Part model, mm, in its own coordinate system. A direction names the side the tool comes from. Round coordinates to 2 decimals unless told otherwise and drop trailing zeros. Write each loop counter-clockwise with the first axis right and the second up, starting at its lowest first coordinate (ties: lowest second). Pieces come first, ordered by that corner, then holes. Notation, with made-up numbers: M 18.5,-7.75 L 52.5,-7.75 A24 ccw 52.5,18.25 Z; hole C 72.5,82 d10. An arc over 180 degrees is marked long. Answer as a JSON object with one key per item and string values. Group by question number.
1. Band-saw the part on A-A, the plane x = 0. Write the cut outline in (y, z).
2. Two-plate mould, pull along Y, no slides. Class faces 1 (the face through (-0.651, 49.957, 6.916)), 2 (the face through (-1.2, -43.8, 13)), 3 (the face through (0, 1, 1)): +Y half, -Y half, draft (parallel to the pull), parting line (faces both ways), or undercut.
3. Drill centre lines: line 1 (Y direction, x = 0.25, z = 9); line 2 (X direction, y = -45, z = 3); line 3 (Y direction, x = -0.5, z = 9). Where is each one in solid material? Low to high. Write a range as from..to.
4. Which spindle directions (+Z, -Z, +X, -X, +Y, -Y) get a long thin tool onto all of the face, cutting with end or side? Do faces 4 (the face through (-0.651, -40.043, 6.916)), 5 (the face through (-0.325, -43.536, 6.409)). Say none if no direction does.
5. Band-saw the part on C-C, the plane z = 4. Write the cut outline in (x, y), plus the area to 3 significant figures.
6. Band-saw the part on B-B, the plane y = -60. Write the cut outline in (x, z), plus the area to 3 significant figures.
7. Drop flat-ended pins along their axis: pin 1 (5 mm diameter, centred on x = -2.5, z = 7, fed in from +Y); pin 2 (5 mm diameter, centred on x = 0.5, z = 4, fed in from -Y). Give the stop position or say it passes through.
8. Band-saw the part on D-D, the plane y = -30. Write the cut outline in (x, z), plus the area to 3 significant figures.
from build123d import *

# Parameters (mm, degrees)
F0_W     = 10
F0_H     = 130
F1_DEPTH = 1
F2_R     = 2
F3_DEPTH = 25
F5_DEPTH = 12
F6_R     = 1.5
F7_DEPTH = 25


with BuildPart() as f1:
    # F0 (on Top) → F1 (new body)
    with BuildSketch(Plane.XY):
        Rectangle(F0_W, F0_H)
    extrude(amount=F1_DEPTH)

    # F2 (on face) → F3 (cut)
    with BuildSketch(Plane.XY.offset(1)):
        with Locations((0, 60)):
            Circle(F2_R)
        with Locations((0, -60)):
            Circle(F2_R)
    extrude(amount=-F3_DEPTH, mode=Mode.SUBTRACT)

    # F4 (on face) → F5 (join)
    with BuildSketch(Plane.XY.offset(1)):
        with BuildLine():
            ThreePointArc((-5, 45), (0, 40), (5, 45))
            ThreePointArc((5, 45), (0, 50), (-5, 45))
        make_face()
        with BuildLine():
            ThreePointArc((-5, -45), (0, -50), (5, -45))
            ThreePointArc((5, -45), (0, -40), (-5, -45))
        make_face()
    extrude(amount=F5_DEPTH)

    # F6 (on face) → F7 (cut)
    with BuildSketch(Plane(origin=(0, 0, 0), x_dir=(1, 0, 0), z_dir=(0, 0, -1))):
        with Locations((0, -45)):
            Circle(F6_R)
        with Locations((0, 45)):
            Circle(F6_R)
    extrude(amount=-F7_DEPTH, mode=Mode.SUBTRACT)


solid = f1.part
Worked answers:
{
 "1": {"outline": "M -65,0 L -62,0 L -62,1 L -65,1 Z; M -58,0 L -46.5,0 L -46.5,13 L -50,13 L -50,1 L -58,1 Z; M -43.5,0 L 43.5,0 L 43.5,13 L 40,13 L 40,1 L -40,1 L -40,13 L -43.5,13 Z; M 46.5,0 L 58,0 L 58,1 L 50,1 L 50,13 L 46.5,13 Z; M 62,0 L 65,0 L 65,1 L 62,1 Z"},
 "2": {"face 1": "undercut", "face 2": "draft", "face 3": "undercut"},
 "3": {"line 1": "y = -49.99..-46.48, -43.52..-40.01, 40.01..43.52, 46.48..49.99", "line 2": "x = -5..-1.5, 1.5..5", "line 3": "y = -49.97..-46.41, -43.59..-40.03, 40.03..43.59, 46.41..49.97"},
 "4": {"face 4": "+Z", "face 5": "+Z, -Z"},
 "5": {"outline": "C 0,-45 d10; C 0,45 d10; hole C 0,-45 d3; hole C 0,45 d3", "area": "143 mm^2"},
 "6": {"outline": "M -5,0 L -2,0 L -2,1 L -5,1 Z; M 2,0 L 5,0 L 5,1 L 2,1 Z", "area": "6.00 mm^2"},
 "7": {"pin 1": "stops at y = 50", "pin 2": "stops at y = -50"},
 "8": {"outline": "M -5,0 L 5,0 L 5,1 L -5,1 Z", "area": "10.0 mm^2"}
}
